```python
from build123d import *


with BuildPart() as f1:
    # F0 (on Front) → F1 (revolve)
    with BuildSketch(Plane.XZ):
        Polygon((0, 2.480038), (0, 0), (4.826, 0), (5.884321, 0.702038), (5.884321, 1.591038), (4.614321, 1.591038), (4.614321, 2.480038), align=None)
        Polygon((-4.826, 0), (0, 0), (0, 2.480038), (-4.614321, 2.480038), (-4.614321, 1.591038), (-5.884321, 1.591038), (-5.884321, 0.702038), align=None)
    revolve(axis=Axis((5.884321, 0, 1.146538), (0, 0, 1)))


solid = f1.part
```
Design review of the part built by this model. Coordinates are the model's own, in mm. A direction names the side the tool comes from. Coordinates: 2 decimals unless noted, no trailing zeros. Use CSV: the item, a comma, the result in double quotes. Start each with the question number.
1) Wall thickness on L1, parallel to X at y = 0, z = 2; L2, parallel to X at y = -2, z = 1.55; L3, parallel to Y at x = -1.5, z = 0.85: over which ranges is each line inside the solid? List them lowest first. Write a range as from..to.
2) For pin 1 Ø3 at (x, y) = (5.5, 6) entering from -Z; pin 2 Ø2 at (x, y) = (5.88, 0) entering from +Z; pin 3 Ø1 at (x, z) = (12, 1) entering from +Y, all flat-tipped, find the tip position at first contact; note any pin that passes through.
3) Tool access review of faces 4 (the conical face through (5.73, 0.06, 0.59)), 5 (the flat face through (6, 0, 1.591)): name each direction out of +Z, -Z, +X, -X, +Y, -Y from which nothing blocks a thin tool from reaching the whole face with its end or side.
4) The part is to be moulded in two halves that separate along Y. For faces 1 (the flat face through (6, 2, 2.48)), 2 (the cylindrical face through (-5.341, -3.535, 1.14)), 3 (the cylindrical face through (7.153, -0.056, 2.042)), say which applies: +Y half, -Y half, draft (parallel to the pull), parting line (faces both ways), or undercut.
Geometry says:
1,L1,"-4.61..4.61, 7.15..16.38"
1,L2,"-5.71..17.48"
1,L3,"-9.16..9.16"
2,pin 1,"z = 0"
2,pin 2,"z = 1.59"
2,pin 3,"y = 10.34"
3,face 4,"-Z"
3,face 5,"+Z"
4,face 1,"draft"
4,face 2,"parting line"
4,face 3,"undercut"
